Here's how the part is built. I have some questions about the finished solid (model axes, mm). Face numbers are marked on the shaded views. A direction names the side the tool comes from. Coordinates: 2 decimals unless noted, no trailing zeros. Write each loop counter-clockwise with the first axis right and the second up, starting at its lowest first coordinate (ties: lowest second). Pieces come first, ordered by that corner, then holes.
Item 1: I'm going to push flat-ended pins straight in: pin 1 Ø10 at (y, z) = (-5.5, 1) entering from +X; pin 2 Ø2.5 at (y, z) = (4.76, -2.75) entering from +X; pin 3 Ø5 at (y, z) = (-4.75, 8.23) entering from +X; pin 4 Ø1.7 at (x, y) = (55.5, 0) entering from -Z. Where does each tip first touch, or does it pass through?
Item 2: For the marked faces 1, 2 and 3, which set-ups out of +Z, -Z, +X, -X, +Y, -Y let a thin tool reach every point of the face, with its end or its side?
Item 3: If we section it at B-B (x = 20.5): Please give me the cut outline in (y, z).
Item 4: If I drill on line 1 (Z direction, x = 1.4, y = 0); line 2 (Y direction, x = 52, z = 0.25); line 3 (Y direction, x = 2.5, z = -3.5), over which ranges is the centre line in solid material (lowest first)?
Item 5: If we section it at A-A (z = -4.5): Please give me the cut outline in (x, y), then the cut area to 3 significant figures.
Item 6: If we section it at D-D (y = -8.25): Please give me the cut outline in (x, z).
Item 7: If we section it at C-C (x = 51.8): Please give me the cut outline in (y, z).
Autodesk Inventor part; units mm, degrees
ref_plane "YZ Plane" through (0, 0, 0) normal (1, 0, 0) x (0, 1, 0)
ref_plane "XZ Plane" through (0, 0, 0) normal (0, 1, 0) x (-1, 0, 0)
ref_plane "XY Plane" through (0, 0, 0) normal (0, 0, 1) x (1, 0, 0)
sketch "スケッチ1" plane through (0, 0, 0) normal (1, 0, 0) x (0, 1, 0)
  circle A0 centre (0, 0) radius 12.2
  dimension "d0" = 24.4
extrude "押し出し1" add sketch "スケッチ1" along normal blind 43.8
sketch "スケッチ2" plane through (43.8, 0, 0) normal (1, 0, 0) x (0, 0, -1)
  circle A0 centre (0, 0) radius 6.5
  dimension "d3" = 13
extrude "押し出し2" add sketch "スケッチ2" along normal blind 2.6
sketch "スケッチ3" plane through (46.4, 0, 0) normal (1, 0, 0) x (0, 0, -1)
  circle A0 centre (0, 0) radius 3
  dimension "d6" = 6
extrude "押し出し3" add sketch "スケッチ3" along normal blind 14.4
sketch "スケッチ4" plane through (60.8, 0, 0) normal (1, 0, 0) x (0, 0, -1)
  circle A0 centre (0, 0) radius 3
  line L0 (2.5, 1.6583) -> (2.5, -1.6583)
  line L1 (0, 0) -> (0, -3)
  dimension "d9" = 6
  dimension "d10" = 2.5
extrude "押し出し4" cut sketch "スケッチ4" against normal blind 11.5 contours A0 L0 picked at (2.5914, -0.3806)
sketch "スケッチ5" plane through (60.8, -1.6583, -2.5) normal (0, 0, -1) x (-1, 0, 0)
  line L0 (0, 0) -> (0, 3.3166)
  point P0 (60.8, 1.6583)
  point P1 (9, 1.6583)
  point P2 (0, 1.6583)
  dimension "d13" = 0
  dimension "d14" = 9
hole "穴1" at (51.8, 0, -2.5) direction (0, 0, 1) diameter 3 end through all
sketch "スケッチ6" plane through (0, 0, 0) normal (-1, 0, 0) x (0, 0, 1)
  arc A0 (-2.5, -1.6583) -> (-2.5, 1.6583) centre (0, 0) ccw
  circle A1 centre (0, 0) radius 3
  point P0 (-2.5, 1.6583)
  dimension "d22" = 6
extrude "押し出し5" add sketch "スケッチ6" along normal blind 4
sketch "スケッチ7" plane through (60.8, 0, 0) normal (1, 0, 0) x (0, 0, -1)
  circle A0 centre (0, 0) radius 6.5
  circle A1 centre (0, 0) radius 1.5
  dimension "d25" = 3
extrude "押し出し6" cut sketch "スケッチ7" against normal blind 6 contours A1
sketch "スケッチ8" plane through (43.8, 0, 0) normal (1, 0, 0) x (0, 0, -1)
  point P0 (0, 0)
  point P1 (0, 9.5)
  point P2 (-8.2272, -4.75)
  point P3 (8.2272, -4.75)
  dimension "d28" = 0
  dimension "d29" = 9.5
  dimension "d32" = 360
hole "穴2" at (43.8, 9.5, 0) at (43.8, -4.75, 8.2272) at (43.8, -4.75, -8.2272) direction (-1, 0, 0) diameter 3 depth 6 tip angle 118
sketch "スケッチ9" plane through (0, 0, 0) normal (-1, 0, 0) x (0, 0, 1)
  point P0 (0, 0)
  point P1 (5.5, 0)
  point P2 (-2.75, 4.7631)
  point P3 (-2.75, -4.7631)
  dimension "d41" = 0
  dimension "d42" = 5.5
  dimension "d45" = 360
hole "穴3" at (0, 0, 5.5) at (0, 4.7631, -2.75) at (0, -4.7631, -2.75) direction (1, 0, 0) diameter 2 depth 6 tip angle 118
properties part number "M2006 P36" material "ステンレス鋼"
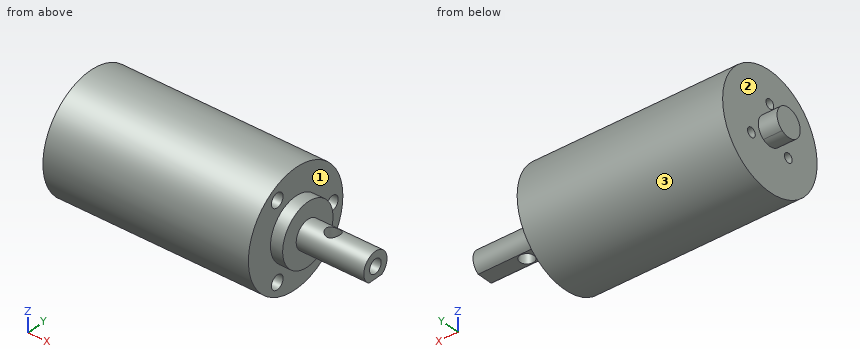
Answer list:
1. pin 1: stops at x = 60.8
1. pin 2: stops at x = 46.4
1. pin 3: stops at x = 43.8
1. pin 4: stops at z = -2.5
2. face 1: +X
2. face 2: -X
2. face 3: +X, -X
3. outline: circle Ø24.4 at (0, 0)
4. line 1: z = -12.2 to 4.5, 6.5 to 12.2
4. line 2: y = -2.99 to -1.49, 1.49 to 2.99
4. line 3: y = -11.69 to -5.42, -4.1 to 4.1, 5.42 to 11.69
5. outline: (0, -11.34) - (43.8, -11.34) - (43.8, -4.69) - (46.4, -4.69) - (46.4, 4.69) - (43.8, 4.69) - (43.8, 11.34) - (0, 11.34) - close
5. area: 1,020 mm2
6. outline: (0, -8.99) - (43.8, -8.99) - (43.8, 8.99) - (0, 8.99) - close
7. outline: (-1.66, -2.5) - (-1.5, -2.5) - (-1.5, 2.6) arc R3 ccw to start; (1.5, -2.5) - (1.66, -2.5) arc R3 ccw to (1.5, 2.6) - close
